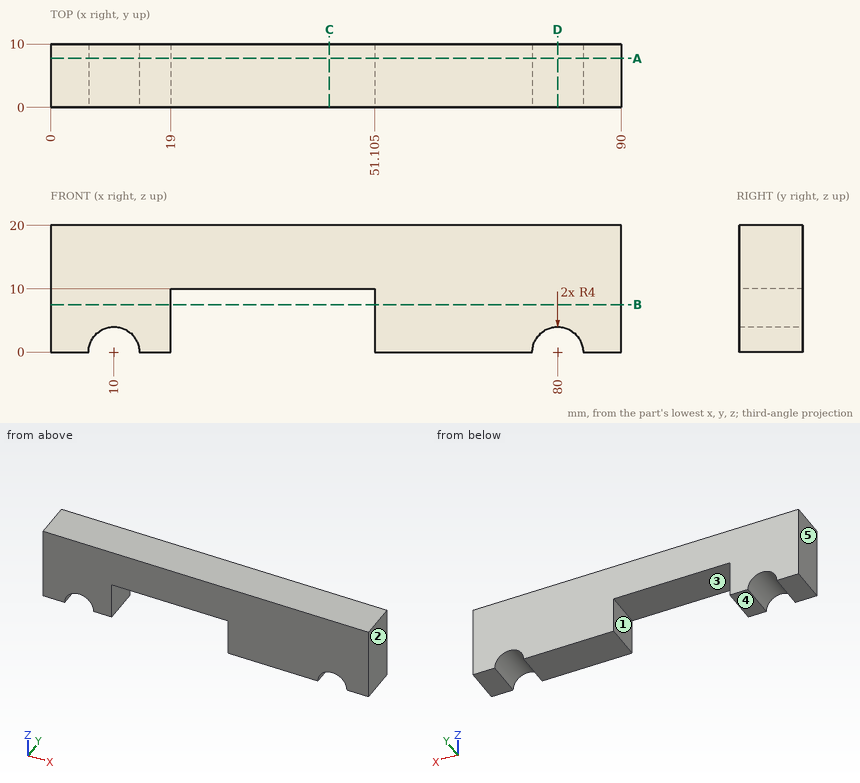
Input: dimensioned drawing with shaded views. Units: mm. Origin: part minimum x, y, z. A direction names the side the tool comes from. Round coordinates to 2 decimals unless told otherwise and drop trailing zeros. Loops run counter-clockwise (first coordinate to the right, second up) from the corner with the lowest first, then second, coordinate; pieces in that order, holes last. Notation, with made-up numbers: M -3.5,33 L 31.5,33 A6 cw 31.5,43 Z; hole C -7.5,-36.75 d3. An arc over 180 degrees is marked long. Return JSON: item names as keys, results as strings. Group by question number.
1. Section query D-D on x = 80. Output: boundary loops of the cut face in (y, z), and give its area (3 significant figures).
2. Section query B-B on z = 7.5. Output: boundary loops of the cut face in (x, y) (1 decimal), and give its area (3 significant figures).
3. Reachability of the marked faces 1 and 2 from +Z, -Z, +X, -X, +Y, -Y: full face, straight path, thin tool, end or side. Return the list, or none.
4. Mould query, pull axis X, two halves, no side actions, for the marked faces 3, 4 and 5. Classes: released by +X, released by -X, zero draft, split by the parting line, or undercut.
5. Section query A-A on y = 7.75. Output: boundary loops of the cut face in (x, z) (1 decimal), and give its area (3 significant figures).
6. Material intervals for line 1 along X through (y, z) = (5, 4.5) (1 decimal); line 2 along Z through (x, y) = (24, 8); line 3 along X through (y, z) = (8.5, 3) (1 decimal), sorted ascending. Write a range as from..to.
7. Section query C-C on x = 44. Output: boundary loops of the cut face in (y, z), and give its area (3 significant figures).
Checks:
{
 "1": {"outline": "M 0,4 L 10,4 L 10,20 L 0,20 Z", "area": "160 mm²"},
 "2": {"outline": "M 0,0 L 19,0 L 19,10 L 0,10 Z; M 51.1,0 L 90,0 L 90,10 L 51.1,10 Z", "area": "579 mm²"},
 "3": {"face 1": "-Z, +Y, -Y", "face 2": "+Z, -Z, +X, +Y, -Y"},
 "4": {"face 3": "undercut", "face 4": "zero draft", "face 5": "released by -X"},
 "5": {"outline": "M 0,0 L 6,0 A4 cw 14,0 L 19,0 L 19,10 L 51.1,10 L 51.1,0 L 76,0 A4 cw 84,0 L 90,0 L 90,20 L 0,20 Z", "area": "1,430 mm²"},
 "6": {"line 1": "x = 0..19, 51.1..90", "line 2": "z = 10..20", "line 3": "x = 0..7.4, 12.6..19, 51.1..77.4, 82.6..90"},
 "7": {"outline": "M 0,10 L 10,10 L 10,20 L 0,20 Z", "area": "100 mm²"}
}
